Geometry: final body of the model. Coordinates: model frame, mm. Face numbers are marked on the shaded views. Give positions to 0.01 mm unless a question says otherwise; leave off trailing zeros. Order: outer loops, then holes, each group sorted by start corner. A loop starts at its lowest first (then second) coordinate and runs counter-clockwise, first axis right, second up. Notation, with made-up numbers: M 13,29 L 28,29 A20 cw 28,66 Z; hole C 88.25,81.25 d2. An arc over 180 degrees is marked long. Write item = value, one per line. Start each with the question number.
Autodesk Inventor part; units mm, degrees
ref_plane "YZ Plane" through (0, 0, 0) normal (1, 0, 0) x (0, 1, 0)
sketch "スケッチ1" plane through (0, 0, 0) normal (0, 0, 1) x (1, 0, 0)
  arc A0 (0, 35) -> (0, -35) centre (0, 0) ccw
  line L0 (0, 35) -> (0, -35)
  dimension "d0" = 70
revolve "回転1" add sketch "スケッチ1" angle 360 about axis through (0, 35, 0) along (0, -1, 0)
sketch "スケッチ2" plane through (0, 0, 0) normal (0, 1, 0) x (-1, 0, 0)
  circle A0 centre (0, 0) radius 20
  dimension "d2" = 40
extrude "押し出し1" cut sketch "スケッチ2" along normal mid plane 100
sketch "スケッチ3" plane through (0, 0, 0) normal (0, 0, 1) x (1, 0, 0)
  circle A0 centre (0, 0) radius 15
  dimension "d5" = 30
extrude "押し出し2" add sketch "スケッチ3" against normal blind 50
properties part number "HandP"
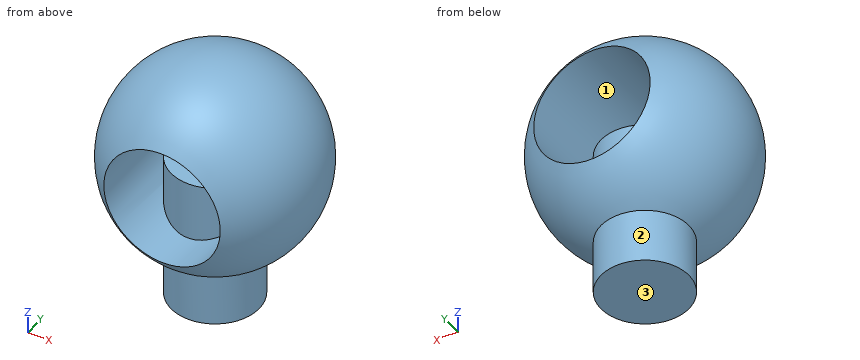
1) Draft query along X for the marked faces 1, 2 and 3. Return one class per face: pulls with the +X half, pulls with the -X half, needs draft (parallel to the pull), parting line crosses it, or undercut.
2) Ray query, L1, parallel to X at y = 20.5, z = -15.5; L2, parallel to X at y = -11, z = -12; L3, parallel to Z at x = 6.5, y = 21. Return the intervals inside material, ascending.
3) Cut plane A-A (x = -9). Return loops of the section in (y, z), plus the area to 3 significant figures.
4) Cut plane C-C (z = 6). Return loops of the section in (x, y), plus the area to 3 significant figures.
5) Cut plane B-B (y = 10). Return loops of the section in (x, z), plus the area to 3 significant figures.
6) Cut plane D-D (x = 16). Return loops of the section in (y, z).
7) Pin query (flat end, axial travel): pin 1 Ø6 at (y, z) = (4.5, -5) entering from +X; pin 2 Ø3 at (y, z) = (-5.5, 3.5) entering from -X; pin 3 Ø10 at (y, z) = (20.5, -9) entering from -X. Return the tip coordinate at first contact, or that it passes through.
Reply:
q1.face_1 = undercut
q1.face_2 = parting line crosses it
q1.face_3 = needs draft
q2.L1 = -23.76 to -12.64, 12.64 to 23.76
q2.L2 = -30.98 to -16, -10.2 to 10.2, 16 to 30.98
q2.L3 = -27.24 to -18.91, 18.91 to 27.24
q3.outline = M -28.72,-17.86 A33.82 ccw -12,-31.62 L -12,-50 L 12,-50 L 12,-31.62 A33.82 ccw 28.72,-17.86 L 12,-17.86 L 12,0 L -12,0 L -12,-17.86 Z; M -28.72,17.86 L 28.72,17.86 A33.82 ccw Z
q3.area = 2,130 mm²
q4.outline = M -19.08,-28.72 L -19.08,28.72 A34.48 ccw Z; M 19.08,-28.72 A34.48 ccw 19.08,28.72 Z
q4.area = 1,250 mm²
q5.outline = M -11.18,-50 L 11.18,-50 L 11.18,-31.62 A33.54 ccw long -11.18,-31.62 Z; hole M -11.18,-16.58 L -11.18,0 L 11.18,0 L 11.18,-16.58 A20 ccw long Z
q5.area = 3,080 mm²
q6.outline = M -28.72,-12 A31.13 ccw 28.72,-12 Z; M -28.72,12 L 28.72,12 A31.13 ccw Z
q7.pin_1 = 34.8
q7.pin_2 = -34.64
q7.pin_3 = -30.37
